from build123d import *

# Parameters (mm, degrees)
SKETCH1_W           = 50
SKETCH1_H           = 50
BOSS_EXTRUDE1_DEPTH = 1.6
SKETCH2_W           = 25
SKETCH2_H           = 3
CUT_EXTRUDE1_DEPTH  = 1.6
FILLET1_R           = 5
FILLET2_R           = 5
FILLET3_R           = 5


with BuildPart() as part:
    # Sketch1 → Boss-Extrude1 (new body)
    with BuildSketch(Plane(origin=(0, 0, 0), x_dir=(1, 0, 0), z_dir=(0, 1, 0))):
        with Locations((25, 25)):
            Rectangle(SKETCH1_W, SKETCH1_H)
    extrude(amount=BOSS_EXTRUDE1_DEPTH)

    # Sketch2 → Cut-Extrude1 (cut)
    with BuildSketch(Plane.XZ):
        with Locations((25, -6.5)):
            Rectangle(SKETCH2_W, SKETCH2_H)
        with Locations((25, -43.5)):
            Rectangle(SKETCH2_W, SKETCH2_H)
    extrude(amount=-CUT_EXTRUDE1_DEPTH, mode=Mode.SUBTRACT)

    # Fillet1
    fillet1_edges = [part.edges().sort_by_distance(p)[0] for p in [
        (0, 0.8, 0),
        (50, 0.8, 0),
    ]]
    fillet(fillet1_edges, radius=FILLET1_R)

    # Fillet2
    fillet2_edges = [part.edges().sort_by_distance(p)[0] for p in [
        (50, 0.8, -50),
    ]]
    fillet(fillet2_edges, radius=FILLET2_R)

    # Fillet3
    fillet3_edges = [part.edges().sort_by_distance(p)[0] for p in [
        (0, 0.8, -50),
    ]]
    fillet(fillet3_edges, radius=FILLET3_R)


solid = part.part
Verification items for the finished model (mm, model axes). A direction names the side the tool comes from. Coordinates: 2 decimals unless noted, no trailing zeros. Order: outer loops, then holes, each group sorted by start corner. A loop starts at its lowest first (then second) coordinate and runs counter-clockwise, first axis right, second up. Notation, with made-up numbers: M 88,-14 L 99,-14 A31 ccw 99,12 Z; hole C -36,73 d6. An arc over 180 degrees is marked long. One line per item, written item: value. Start each with the question number.
Item 1: Mould release check, pull along X, two halves, no side actions. Record for faces 1 (the flat face through (50, 1, -25)), 2 (the flat face through (37.5, 1, -7)), 3 (the flat face through (25, 1, -50)): pulls with the +X half, pulls with the -X half, needs draft (parallel to the pull), parting line crosses it, or undercut.
Item 2: Thickness scan on probe 1 along Z at (x, y) = (18.5, 0.35); probe 2 along X at (y, z) = (0.4, -5.5); probe 3 along Z at (x, y) = (4.5, 1). Record the ranges inside material, lowest first.
Item 3: Sectioned sample at C-C on x = 36.5. Record the cut outline in (y, z).
Item 4: Sectioned sample at A-A on y = 0.8. Record the cut outline in (x, z).
Item 5: Access from +Z, -Z, +X, -X, +Y, -Y to the whole of each face (thin tool, end or side, straight path). Record for faces 4 (the flat face through (25, 0, -25)), 5 (the flat face through (25, 1, -42)).
Item 6: Sectioned sample at B-B on z = -44. Record the cut outline in (x, y).
Calculated:
1. face 1: pulls with the +X half
1. face 2: undercut
1. face 3: needs draft
2. probe 1: -50 to -45, -42 to -8, -5 to 0
2. probe 2: 0 to 12.5, 37.5 to 50
2. probe 3: -49.97 to -0.03
3. outline: M 0,-50 L 1.6,-50 L 1.6,-45 L 0,-45 Z; M 0,-42 L 1.6,-42 L 1.6,-8 L 0,-8 Z; M 0,-5 L 1.6,-5 L 1.6,0 L 0,0 Z
4. outline: M 0,-45 A5 ccw 5,-50 L 45,-50 A5 ccw 50,-45 L 50,-5 A5 ccw 45,0 L 5,0 A5 ccw 0,-5 Z; hole M 12.5,-45 L 37.5,-45 L 37.5,-42 L 12.5,-42 Z; hole M 12.5,-8 L 37.5,-8 L 37.5,-5 L 12.5,-5 Z
5. face 4: +Z, -Z, +X, -X, -Y
5. face 5: +Y, -Y
6. outline: M 0,0 L 12.5,0 L 12.5,1.6 L 0,1.6 Z; M 37.5,0 L 50,0 L 50,1.6 L 37.5,1.6 Z
